from build123d import *

# Parameters (mm, degrees)
SKETCH1_W           = 15.135
SKETCH1_H           = 12.5
BASE_DEPTH          = 5
SKETCH2_W           = 15.135
SKETCH2_H           = 15
BOSS_EXTRUDE2_DEPTH = 1.5
BOSS_EXTRUDE3_DEPTH = 15.135
SKETCH4_W           = 9.135
SKETCH4_H           = 15
CUT_EXTRUDE1_DEPTH  = 11
SKETCH5_R           = 1.375
CUT_EXTRUDE2_DEPTH  = 2
SKETCH6_R           = 1.375
CUT_EXTRUDE3_DEPTH  = 5.75
CUT_EXTRUDE4_DEPTH  = 25.485172511


with BuildPart() as part:
    # Sketch1 → base (new body)
    with BuildSketch(Plane(origin=(0, 0, 0), x_dir=(1, 0, 0), z_dir=(0, 1, 0))):
        with Locations((7.5675, 6.25)):
            Rectangle(SKETCH1_W, SKETCH1_H)
    extrude(amount=BASE_DEPTH)

    # Sketch2 → Boss-Extrude2 (add)
    with BuildSketch(Plane(origin=(0, 0, -12.5), x_dir=(-1, 0, 0), z_dir=(0, 0, -1))):
        with Locations((-7.5675, -7.5)):
            Rectangle(SKETCH2_W, SKETCH2_H)
    extrude(amount=-BOSS_EXTRUDE2_DEPTH)

    # Sketch3 → Boss-Extrude3 (add)
    with BuildSketch(Plane.ZY):
        Polygon((0, 0), (-11, -15), (-11, 0), align=None)
    extrude(amount=-BOSS_EXTRUDE3_DEPTH)

    # Sketch4 → Cut-Extrude1 (cut)
    with BuildSketch(Plane.XY):
        with Locations((7.5675, -7.5)):
            Rectangle(SKETCH4_W, SKETCH4_H)
    extrude(amount=-CUT_EXTRUDE1_DEPTH, mode=Mode.SUBTRACT)

    # Sketch5 → Cut-Extrude2 (cut)
    with BuildSketch(Plane.XY.offset(-11)):
        with Locations((7.5675, -4)):
            Circle(SKETCH5_R)
        with Locations((7.5675, -11)):
            Circle(SKETCH5_R)
    extrude(amount=-CUT_EXTRUDE2_DEPTH, mode=Mode.SUBTRACT)

    # Sketch6 → Cut-Extrude3 (cut)
    with BuildSketch(Plane(origin=(0, 5, 0), x_dir=(1, 0, 0), z_dir=(0, 1, 0))):
        with Locations((6.5675, 6.25)):
            Circle(SKETCH6_R)
    extrude(amount=-CUT_EXTRUDE3_DEPTH, mode=Mode.SUBTRACT)

    # Sketch7 → Cut-Extrude4 (cut)
    with BuildSketch(Plane.ZY.offset(-12.135)):
        Polygon((-11, -15), (0, 0), (-11, 0), align=None)
    extrude(amount=CUT_EXTRUDE4_DEPTH, mode=Mode.SUBTRACT)


solid = part.part
The model under review builds one solid part; all positions refer to its coordinate system, in mm. A direction names the side the tool comes from. Round coordinates to 2 decimals unless told otherwise and drop trailing zeros. Loops run counter-clockwise (first coordinate to the right, second up) from the corner with the lowest first, then second, coordinate; pieces in that order, holes last. Notation, with made-up numbers: M -4,56 L 44,56 A28 ccw 44,81 Z; hole C -36,12 d2. An arc over 180 degrees is marked long. Answer as CSV lines item,"result".
1. We need section C-C (x = 13.5). Give the boundary of the cut face in (y, z), plus the area to 4 significant figures.
Outcome:
outline,"M -15,-12.5 L 5,-12.5 L 5,0 L 0,0 L -15,-11 Z"
area,"167.5 mm2"
2. We need section B-B (y = -4.75). Give the boundary of the cut face in (x, z) (3 decimals).
Outcome:
outline,"M 0,-12.5 L 6.415,-12.5 L 6.415,-11 L 0,-11 Z; M 8.72,-12.5 L 15.135,-12.5 L 15.135,-3.483 L 12.135,-3.483 L 12.135,-11 L 8.72,-11 Z"
3. Insertion check: pin 1 Ø3 at (x, y) = (7.57, -11) entering from +Z; pin 2 Ø5.5 at (x, z) = (9, -4) entering from -Y; pin 3 Ø3 at (x, y) = (7.57, -4) entering from -Z; pin 4 Ø5 at (x, y) = (10, -8.5) entering from +Z. Each pin has a flat end and moves straight along its axis. Give the tip position at first contact, or say it passes through.
Outcome:
pin 1,"stops at z = -11"
pin 2,"stops at y = 0"
pin 3,"stops at z = -12.5"
pin 4,"stops at z = -5.28"
4. We need section A-A (z = -6.25). Give the boundary of the cut face in (x, y) (1 decimal), plus the area to 3 significant figures.
Outcome:
outline,"M 0,0 L 5.2,0 L 5.2,5 L 0,5 Z; M 7.9,0 L 12.1,0 L 12.1,-8.5 L 15.1,-8.5 L 15.1,5 L 7.9,5 Z"
area,"87.5 mm2"
5. To check wall thickness, follow L1, parallel to X at y = -1, z = -9.5 (3 decimals); L2, parallel to Y at x = 4.25, z = -4.25; L3, parallel to Z at x = 7.5, y = 4. State the ranges of each line that lie inside material, in increasing order. Write a range as [from, to].
Outcome:
L1,"x = [12.135, 15.135]"
L2,"y = [0, 5]"
L3,"z = [-12.5, -7.26], [-5.24, 0]"
6. For faces 1 (the face through (7, 2, 0)), 2 (the face through (6, -7, -11)), list the 3-axis set-ups (+Z, -Z, +X, -X, +Y, -Y) from which the entire face can be reached by the end or side of a thin tool; tool diameter is ignored.
Outcome:
face 1,"+Z, +X, -X, +Y, -Y"
face 2,"+Z, -X, -Y"
7. Draft analysis for pull direction Y (two halves, no side actions). For faces 3 (the face through (7, 5, -8)), 4 (the face through (13.614, -7.395, -5.423)), 5 (the face through (6.48, -4.84, -11.74)), state which applies: pulls with the +Y half, pulls with the -Y half, needs draft (parallel to the pull), parting line crosses it, or undercut.
Outcome:
face 3,"pulls with the +Y half"
face 4,"pulls with the -Y half"
face 5,"undercut"
